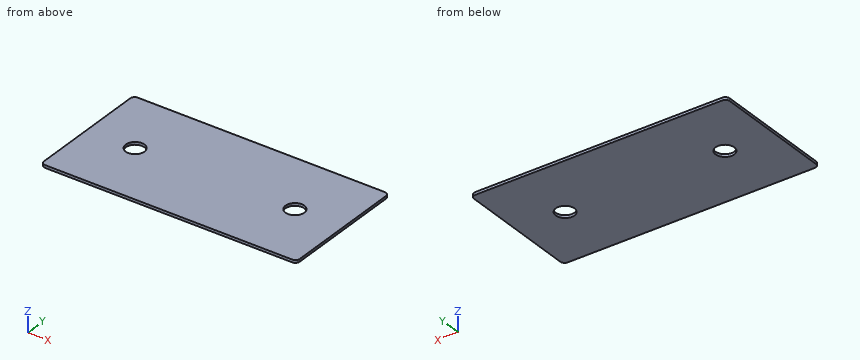
from build123d import *

# Parameters (mm, degrees)
F0_R     = 11.176
F1_DEPTH = 1.5875


with BuildPart() as f1:
    # F0 (on Top) → F1 (new body, symmetric)
    with BuildSketch(Plane.XY):
        with BuildLine():
            ThreePointArc((-147.32, 76.2), (-150.9121024484, 74.7121024484), (-152.4, 71.12))
            Line((-152.4, 71.12), (-152.4, -71.12))
            ThreePointArc((-152.4, -71.12), (-150.9121024484, -74.7121024484), (-147.32, -76.2))
            Line((-147.32, -76.2), (147.32, -76.2))
            ThreePointArc((147.32, -76.2), (150.9121024484, -74.7121024484), (152.4, -71.12))
            Line((152.4, -71.12), (152.4, 71.12))
            ThreePointArc((152.4, 71.12), (150.9121024484, 74.7121024484), (147.32, 76.2))
            Line((147.32, 76.2), (-147.32, 76.2))
        make_face()
        with Locations((-95.25, 0)):
            Circle(F0_R, mode=Mode.SUBTRACT)
        with Locations((95.25, 0)):
            Circle(F0_R, mode=Mode.SUBTRACT)
    extrude(amount=F1_DEPTH, both=True)


solid = f1.part
Check sheet for the modelled part. Datum: model origin and axes. Units: mm. Round coordinates to 2 decimals unless told otherwise and drop trailing zeros. Write each loop counter-clockwise with the first axis right and the second up, starting at its lowest first coordinate (ties: lowest second). Pieces come first, ordered by that corner, then holes. Notation, with made-up numbers: (-13.75, 34) - (39.25, 34) arc R27 cw to (39.25, 59) - close; hole circle Ø1 at (-13.5, -21.5). An arc over 180 degrees is marked (long way). Return JSON: item names as keys, results as strings.
Q1. Cross-section at A-A (y = 0). Record the boundary of the cut face in (x, z).
Returned:
{"outline": "(-152.4, -1.59) - (-106.43, -1.59) - (-106.43, 1.59) - (-152.4, 1.59) - close; (-84.07, -1.59) - (84.07, -1.59) - (84.07, 1.59) - (-84.07, 1.59) - close; (106.43, -1.59) - (152.4, -1.59) - (152.4, 1.59) - (106.43, 1.59) - close"}
Q2. Scan lines: L1, parallel to X at y = 0.5, z = 1; L2, parallel to Y at x = -95.25, z = -0.1; L3, parallel to X at y = 7.5, z = -1.3. Record each from-to range of solid material in increasing order. Write a range as from..to.
Returned:
{"L1": "x = -152.4..-106.41, -84.09..84.09, 106.41..152.4", "L2": "y = -76.2..-11.18, 11.18..76.2", "L3": "x = -152.4..-103.54, -86.96..86.96, 103.54..152.4"}
Q3. Depth check by flat-ended pin: P1, Ø13.5, axis at x = -95.25, y = 0, coming from the +Z side. Enter the tip coordinate at first touch or a pass-through.
Returned:
{"P1": "passes through"}
Q4. Cross-section at B-B (x = -95.25). Record the boundary of the cut face in (y, z).
Returned:
{"outline": "(-76.2, -1.59) - (-11.18, -1.59) - (-11.18, 1.59) - (-76.2, 1.59) - close; (11.18, -1.59) - (76.2, -1.59) - (76.2, 1.59) - (11.18, 1.59) - close"}
Q5. Cross-section at C-C (z = -0.2). Record the boundary of the cut face in (x, y), then the cut area to 3 significant figures.
Returned:
{"outline": "(-152.4, -71.12) arc R5.08 ccw to (-147.32, -76.2) - (147.32, -76.2) arc R5.08 ccw to (152.4, -71.12) - (152.4, 71.12) arc R5.08 ccw to (147.32, 76.2) - (-147.32, 76.2) arc R5.08 ccw to (-152.4, 71.12) - close; hole circle Ø22.35 at (-95.25, 0); hole circle Ø22.35 at (95.25, 0)", "area": "45,600 mm²"}
